Could you check a few things on this model? Use its own coordinates, in mm. Coordinates: 2 decimals unless noted, no trailing zeros. Write each loop counter-clockwise with the first axis right and the second up, starting at its lowest first coordinate (ties: lowest second). Pieces come first, ordered by that corner, then holes. Notation, with made-up numbers: (-13, -28.5) - (37, -28.5) arc R20 ccw to (37, -9.5) - close; hole circle Ø8 at (-10.75, -3.5). An arc over 180 degrees is marked (long way). Answer as a JSON object with one key per item and string values. Group by question number.
1) Will this pin go through, and if not, where does the flat tip stop? pin 1 Ø2 at (y, z) = (-2, 1.5) entering from +X.
2) Please list where these lines run through material, in increasing order: line 1 along Y through (x, z) = (48, 0.05); line 2 along X through (y, z) = (-0.4, 1.7); line 3 along X through (y, z) = (-0.65, 1.6).
3) If we section it at A-A (y = 0): Write out the boundary of the cut face in (x, z), plus the area to 3 significant figures.
4) If we section it at B-B (z = -0.5): Write out the boundary of the cut face in (x, y), plus the area to 3 significant figures.
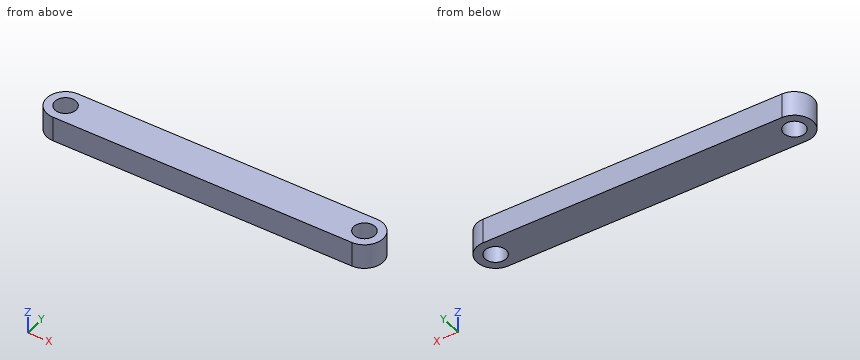
Autodesk Inventor part; units mm, degrees
ref_plane "YZ Plane" through (0, 0, 0) normal (1, 0, 0) x (0, 1, 0)
ref_plane "XZ Plane" through (0, 0, 0) normal (0, 1, 0) x (-1, 0, 0)
ref_plane "XY Plane" through (0, 0, 0) normal (0, 0, 1) x (1, 0, 0)
sketch "スケッチ1" plane through (0, 0, 0) normal (0, 0, 1) x (1, 0, 0)
  circle A0 centre (0, 0) radius 1.7
  circle A1 centre (48, 0) radius 1.7
  circle A2 centre (0, 0) radius 3
  circle A3 centre (48, 0) radius 3
  line L0 (0, 3) -> (48, 3)
  line L1 (0, -3) -> (48, -3)
  dimension "d0" = 3.4
  dimension "d1" = 3.4
  dimension "d2" = 6
  dimension "d3" = 6
  dimension "d4" = 48
extrude "押し出し1" add sketch "スケッチ1" along normal mid plane 4
properties part number "HbFingerMainCouplerLink01"
Here are the results:
{
 "1": {"pin 1": "stops at x = 50.83"},
 "2": {"line 1": "y = -3 to -1.7, 1.7 to 3", "line 2": "x = -2.97 to -1.65, 1.65 to 46.35, 49.65 to 50.97", "line 3": "x = -2.93 to -1.57, 1.57 to 46.43, 49.57 to 50.93"},
 "3": {"outline": "(-3, -2) - (-1.7, -2) - (-1.7, 2) - (-3, 2) - close; (1.7, -2) - (46.3, -2) - (46.3, 2) - (1.7, 2) - close; (49.7, -2) - (51, -2) - (51, 2) - (49.7, 2) - close", "area": "189 mm²"},
 "4": {"outline": "(0, -3) - (48, -3) arc R3 ccw to (48, 3) - (0, 3) arc R3 ccw to start; hole circle Ø3.4 at (0, 0); hole circle Ø3.4 at (48, 0)", "area": "298 mm²"}
}
